from build123d import *

# Parameters (mm, degrees)
SKETCH_1_R          = 1.5
EXTRUDE_1_DEPTH     = 3
CHAMFER_1_SIZE      = 7
FILLET_1_R          = 5
SKETCH_2_W          = 70
SKETCH_2_H          = 20
EXTRUDE_2_DEPTH     = 3
SKETCH_3_R          = 2
CUT_EXTRUDE_1_DEPTH = 3
FILLET_2_R          = 5


with BuildPart() as part:
    # 草图1 → 凸台-拉伸1 (new body)
    with BuildSketch(Plane(origin=(0, 0, 0), x_dir=(1, 0, 0), z_dir=(0, 1, 0))):
        Polygon((-55, 50), (-55, -50), (55, -50), (55, 50), (40, 50), (40, 95), (-40, 95), (-40, 50), align=None)
        with Locations(Location((-43.343145751, -44, 0), (0, 0, 270))):
            Circle(SKETCH_1_R, mode=Mode.SUBTRACT)
        with Locations(Location((-49, -38.343145751, 0), (0, 0, 270))):
            Circle(SKETCH_1_R, mode=Mode.SUBTRACT)
        with Locations(Location((43.343145751, -44, 0), (0, 0, 270))):
            Circle(SKETCH_1_R, mode=Mode.SUBTRACT)
        with Locations(Location((49, -38.343145751, 0), (0, 0, 270))):
            Circle(SKETCH_1_R, mode=Mode.SUBTRACT)
        with Locations(Location((-49, 38.343145751, 0), (0, 0, 270))):
            Circle(SKETCH_1_R, mode=Mode.SUBTRACT)
        with Locations(Location((-43.343145751, 44, 0), (0, 0, 270))):
            Circle(SKETCH_1_R, mode=Mode.SUBTRACT)
        with Locations(Location((49, 38.343145751, 0), (0, 0, 270))):
            Circle(SKETCH_1_R, mode=Mode.SUBTRACT)
        with Locations(Location((43.343145751, 44, 0), (0, 0, 270))):
            Circle(SKETCH_1_R, mode=Mode.SUBTRACT)
        with Locations(Location((35, 85, 0), (0, 0, 270))):
            Circle(SKETCH_1_R, mode=Mode.SUBTRACT)
        with Locations(Location((-35, 85, 0), (0, 0, 270))):
            Circle(SKETCH_1_R, mode=Mode.SUBTRACT)
    extrude(amount=EXTRUDE_1_DEPTH)

    # 倒角1
    chamfer_1_edges = [part.edges().sort_by_distance(p)[0] for p in [
        (-55, 1.5, 50),
        (-55, 1.5, -50),
        (55, 1.5, -50),
        (55, 1.5, 50),
    ]]
    chamfer(chamfer_1_edges, length=CHAMFER_1_SIZE)

    # 圆角1
    fillet_1_edges = [part.edges().sort_by_distance(p)[0] for p in [
        (-40, 1.5, -50),
        (-40, 1.5, -95),
        (40, 1.5, -95),
        (40, 1.5, -50),
    ]]
    fillet(fillet_1_edges, radius=FILLET_1_R)

    # 草图2 → 凸台-拉伸2 (add)
    with BuildSketch(Plane(origin=(0, 3, 0), x_dir=(1, 0, 0), z_dir=(0, 1, 0))):
        with Locations((0, -60)):
            Rectangle(SKETCH_2_W, SKETCH_2_H)
    extrude(amount=-EXTRUDE_2_DEPTH)

    # 草图3 → 切除-拉伸1 (cut)
    with BuildSketch(Plane(origin=(0, 3, 0), x_dir=(1, 0, 0), z_dir=(0, 1, 0))):
        with Locations(Location((-40.14, 29.5, 0), (0, 0, 270))):
            Circle(SKETCH_3_R)
        with Locations(Location((44.86, 27, 0), (0, 0, 270))):
            Circle(SKETCH_3_R)
        with Locations(Location((-29.14, -49, 0), (0, 0, 270))):
            Circle(SKETCH_3_R)
        with Locations(Location((28.86, -49, 0), (0, 0, 270))):
            Circle(SKETCH_3_R)
        with Locations(Location((8.86, 33, 0), (0, 0, 270))):
            Circle(SKETCH_3_R)
    extrude(amount=-CUT_EXTRUDE_1_DEPTH, mode=Mode.SUBTRACT)

    # 圆角2
    fillet_2_edges = [part.edges().sort_by_distance(p)[0] for p in [
        (-35, 1.5, 70),
        (-35, 1.5, 50),
        (35, 1.5, 50),
        (35, 1.5, 70),
    ]]
    fillet(fillet_2_edges, radius=FILLET_2_R)


solid = part.part
Here's how the part is built. I have some questions about the finished solid (model axes, mm). A direction names the side the tool comes from. Coordinates: 2 decimals unless noted, no trailing zeros. Write each loop counter-clockwise with the first axis right and the second up, starting at its lowest first coordinate (ties: lowest second). Pieces come first, ordered by that corner, then holes. Notation, with made-up numbers: (66, -11) - (111, -11) arc R19 cw to (111, 26) - close; hole circle Ø1 at (65.5, 54.25). An arc over 180 degrees is marked (long way). Use one line per item in the form item = value.
1) On a 3-axis mill with a long thin cutter (end or side, diameter ignored), from which of +Z, -Z, +X, -X, +Y, -Y can I reach the whole of each face in a straight line? I mean faces 5 (the flat face through (40, 1, -72)), 6 (the flat face through (55, 1, 1)), 7 (the flat face through (44, 1, 50)). Say none if no direction works.
Solved:
face_5 = -Z, +X, +Y, -Y
face_6 = +Z, -Z, +X, +Y, -Y
face_7 = +Z, +X, +Y, -Y
2) Thinking about a two-plate mould opening in X: for faces 1 (the cylindrical face through (-36.33, 1.48, -84.31)), 2 (the flat face through (-51, 1, -47)), 3 (the flat face through (-46, 1, -50)), 4 (the cylindrical face through (33, 1, 69)), which applies, released by +X, released by -X, zero draft, split by the parting line, or undercut?
Solved:
face_1 = undercut
face_2 = released by -X
face_3 = zero draft
face_4 = released by +X
3) I need wall thicknesses on line 1 (X direction, y = 0.35, z = -39.5); line 2 (X direction, y = 2.4, z = 39); line 3 (Z direction, x = -48, y = 2.15). Which ranges of each line are inside material? Lowest first, please.
Solved:
line_1 = -55 to -49.95, -48.05 to 48.05, 49.95 to 55
line_2 = -55 to -50.35, -47.65 to 47.65, 50.35 to 55
line_3 = -50 to -39.46, -37.23 to 37.23, 39.46 to 50
4) Suppose I cut it at B-B, the plane z = -52. Write out the boundary of the cut face in (x, y), plus the area to 3 significant figures.
Solved:
outline = (-41, 0) - (41, 0) - (41, 3) - (-41, 3) - close
area = 246 mm2
5) I'm going to push flat-ended pins straight in: P1, Ø1.5, axis at x = -46, y = 1, coming from the -Z side; P2, Ø0.9, axis at y = 1, z = 61, coming from the +X side. Where does each tip first touch, or does it pass through?
Solved:
P1 = -50
P2 = 35
6) Suppose I cut it at A-A, the plane y = 1.15. Give the number of separate pieces and of enclosed holes in the cut face, plus the area to 3 significant figures.
Solved:
separate_pieces = 1
enclosed_holes = 15
area = 15,800 mm2
